Check sheet for the modelled part. Datum: model origin and axes. Units: mm. Round coordinates to 2 decimals unless told otherwise and drop trailing zeros. Order: outer loops, then holes, each group sorted by start corner. A loop starts at its lowest first (then second) coordinate and runs counter-clockwise, first axis right, second up.
Q1. Cross-section at A-A on y = -12. Record the cut outline in (x, z), then the cut area to 3 significant figures.
Q2. Cross-section at D-D on y = -17.5. Record the cut outline in (x, z).
Q3. Cross-section at C-C on x = 15. Record the cut outline in (y, z), then the cut area to 3 significant figures.
Q4. Cross-section at B-B on z = 10.04. Record the cut outline in (x, y), then the cut area to 3 significant figures.
Q5. Mould release check, pull along Z, two halves, no side actions. Record for faces 1 (the cylindrical face through (17.194, -11.832, 7.787)), 2 (the cylindrical face through (9.9, -11.13, 23.67)), 3 (the flat face through (10, -12, 0)), 4 (the flat face through (20.08, -12, 20)): +Z half, -Z half, draft (parallel to the pull), parting line (faces both ways), or undercut.
Q6. Scan lines: probe 1 along Z at (x, y) = (10.04, -12); probe 2 along Z at (x, y) = (5.25, -12); probe 3 along X at (y, z) = (-11.25, 10.5). Record each from-to range of solid material in increasing order.
from build123d import *

# Parameters (mm, degrees)
F1_DEPTH = 24
F2_R     = 4
F3_DEPTH = 25.4
F4_SIZE  = 3.81


with BuildPart() as f1:
    # F0 (on Front) → F1 (new body)
    with BuildSketch(Plane.XZ):
        with BuildLine():
            Line((0, 37.6314), (0, 0))
            Line((0, 0), (10.04, 0))
            Line((10.04, 0), (10.04, 2.54))
            ThreePointArc((10.04, 2.54), (2.54, 10.04), (10.04, 17.54))
            ThreePointArc((10.04, 17.54), (15.3433008589, 15.3433008589), (17.54, 10.04))
            Line((17.54, 10.04), (20.08, 10.04))
            Line((20.08, 10.04), (20.08, 37.6314))
            Line((20.08, 37.6314), (0, 37.6314))
        make_face()
        with BuildLine():
            ThreePointArc((17.5457, 27.5857), (15.3473313676, 22.2783686324), (10.04, 20.08))
            ThreePointArc((10.04, 20.08), (4.7326686324, 32.8930313676), (17.5457, 27.5857))
        make_face(mode=Mode.SUBTRACT)
        with BuildLine():
            ThreePointArc((17.5457, 27.5857), (4.7326686324, 32.8930313676), (10.04, 20.08))
            ThreePointArc((10.04, 20.08), (15.3473313676, 22.2783686324), (17.5457, 27.5857))
        make_face()
        with BuildLine():
            ThreePointArc((14.04, 27.5857), (12.8684271247, 24.7572728753), (10.04, 23.5857))
            ThreePointArc((10.04, 23.5857), (7.2115728753, 30.4141271247), (14.04, 27.5857))
        make_face(mode=Mode.SUBTRACT)
        with BuildLine():
            Line((10.04, 2.54), (10.04, 0))
            Line((10.04, 0), (20.08, 0))
            Line((20.08, 0), (20.08, 10.04))
            Line((20.08, 10.04), (17.54, 10.04))
            ThreePointArc((17.54, 10.04), (15.3433008589, 4.7366991411), (10.04, 2.54))
        make_face()
        with BuildLine():
            ThreePointArc((14.04, 27.5857), (7.2115728753, 30.4141271247), (10.04, 23.5857))
            ThreePointArc((10.04, 23.5857), (12.8684271247, 24.7572728753), (14.04, 27.5857))
        make_face()
    extrude(amount=F1_DEPTH)

    # F2 (on face) → F3 (cut)
    with BuildSketch(Plane(origin=(0, 0, 0), x_dir=(0, -1, 0), z_dir=(-1, 0, 0))):
        with Locations((12, 27.573)):
            Circle(F2_R)
    extrude(amount=-F3_DEPTH, mode=Mode.SUBTRACT)

    # F4
    f4_edges = [f1.edges().sort_by_distance(p)[0] for p in [
        (10.04, 0, 37.6314),
        (0, -12, 0),
        (10.04, -24, 37.6314),
        (20.08, -12, 0),
    ]]
    chamfer(f4_edges, length=F4_SIZE)


solid = f1.part
Results found:
1. outline: (0, 3.81) - (3.81, 0) - (16.27, 0) - (20.08, 3.81) - (20.08, 23.57) - (0, 23.57) - close; (0, 31.57) - (20.08, 31.57) - (20.08, 37.63) - (0, 37.63) - close; hole circle Ø15 at (10.04, 10.04)
1. area: 404 mm2
2. outline: (0, 3.81) - (3.81, 0) - (16.27, 0) - (20.08, 3.81) - (20.08, 37.63) - (0, 37.63) - close; hole circle Ø15 at (10.04, 10.04)
3. outline: (-24, 0) - (0, 0) - (0, 4.41) - (-24, 4.41) - close; (-24, 15.67) - (0, 15.67) - (0, 33.82) - (-3.81, 37.63) - (-20.19, 37.63) - (-24, 33.82) - close; hole circle Ø8 at (-12, 27.57)
3. area: 568 mm2
4. outline: (0, -24) - (2.54, -24) - (2.54, 0) - (0, 0) - close; (17.54, -24) - (20.08, -24) - (20.08, 0) - (17.54, 0) - close
4. area: 122 mm2
5. face 1: undercut
5. face 2: undercut
5. face 3: -Z half
5. face 4: draft
6. probe 1: z = 0 to 2.54, 17.54 to 23.57, 31.57 to 37.63
6. probe 2: z = 0 to 4.27, 15.81 to 23.57, 31.57 to 37.63
6. probe 3: x = 0 to 2.55, 17.53 to 20.08
